```python
from build123d import *

# Parameters (mm, degrees)
F1_DEPTH = 15
F2_DEPTH = 3
F3_DEPTH = 50
F4_DEPTH = 53


with BuildPart() as f1:
    # F0 (on Top) → F1 (new body)
    with BuildSketch(Plane.XY):
        with BuildLine():
            Line((37.5, -20), (37.5, 30))
            Line((37.5, 30), (-27.5, 30))
            Line((-27.5, 30), (-27.5, 26))
            ThreePointArc((-27.5, 26), (-23.2573593129, 24.2426406871), (-21.5, 20))
            ThreePointArc((-21.5, 20), (-27.5, 14), (-33.5, 20))
            Line((-33.5, 20), (-37.5, 20))
            Line((-37.5, 20), (-37.5, -30))
            Line((-37.5, -30), (27.5, -30))
            Line((27.5, -30), (27.5, -26))
            ThreePointArc((27.5, -26), (23.2573593129, -15.7573593129), (33.5, -20))
            Line((33.5, -20), (37.5, -20))
        make_face()
        with BuildLine():
            ThreePointArc((-19, -19.25), (-27.5355339059, -22.7855339059), (-24, -14.25))
            ThreePointArc((-24, -14.25), (-20.4644660941, -15.7144660941), (-19, -19.25))
        make_face(mode=Mode.SUBTRACT)
        with BuildLine():
            ThreePointArc((25.05, -6.2), (16.5144660941, -9.7355339059), (20.05, -1.2))
            ThreePointArc((20.05, -1.2), (23.5855339059, -2.6644660941), (25.05, -6.2))
        make_face(mode=Mode.SUBTRACT)
        with BuildLine():
            ThreePointArc((5, 19.35), (3.5355339059, 15.8144660941), (0, 14.35))
            ThreePointArc((0, 14.35), (-3.5355339059, 22.8855339059), (5, 19.35))
        make_face(mode=Mode.SUBTRACT)
        with BuildLine():
            Line((-27.5, 26), (-27.5, 30))
            Line((-27.5, 30), (-37.5, 30))
            Line((-37.5, 30), (-37.5, 20))
            Line((-37.5, 20), (-33.5, 20))
            ThreePointArc((-33.5, 20), (-31.7426406871, 24.2426406871), (-27.5, 26))
        make_face()
        with BuildLine():
            Line((37.5, -30), (37.5, -20))
            Line((37.5, -20), (33.5, -20))
            ThreePointArc((33.5, -20), (31.7426406871, -24.2426406871), (27.5, -26))
            Line((27.5, -26), (27.5, -30))
            Line((27.5, -30), (37.5, -30))
        make_face()
    extrude(amount=F1_DEPTH)

    # F0 (on Top) → F2 (join)
    with BuildSketch(Plane.XY):
        with BuildLine():
            ThreePointArc((-21.5, 20), (-23.2573593129, 24.2426406871), (-27.5, 26))
            Line((-27.5, 26), (-27.5, 22))
            ThreePointArc((-27.5, 22), (-26.0857864376, 21.4142135624), (-25.5, 20))
            ThreePointArc((-25.5, 20), (-27.5, 18), (-29.5, 20))
            Line((-29.5, 20), (-33.5, 20))
            ThreePointArc((-33.5, 20), (-27.5, 14), (-21.5, 20))
        make_face()
        with BuildLine():
            Line((-27.5, 22), (-27.5, 26))
            ThreePointArc((-27.5, 26), (-31.7426406871, 24.2426406871), (-33.5, 20))
            Line((-33.5, 20), (-29.5, 20))
            ThreePointArc((-29.5, 20), (-28.9142135624, 21.4142135624), (-27.5, 22))
        make_face()
        with BuildLine():
            ThreePointArc((27.5, -26), (31.7426406871, -24.2426406871), (33.5, -20))
            Line((33.5, -20), (29.5, -20))
            ThreePointArc((29.5, -20), (28.9142135624, -21.4142135624), (27.5, -22))
            Line((27.5, -22), (27.5, -26))
        make_face()
        with BuildLine():
            Line((29.5, -20), (33.5, -20))
            ThreePointArc((33.5, -20), (23.2573593129, -15.7573593129), (27.5, -26))
            Line((27.5, -26), (27.5, -22))
            ThreePointArc((27.5, -22), (26.0857864376, -18.5857864376), (29.5, -20))
        make_face()
    extrude(amount=F2_DEPTH)

    # F0 (on Top) → F3 (join)
    with BuildSketch(Plane.XY):
        with BuildLine():
            ThreePointArc((5, 19.35), (-3.5355339059, 22.8855339059), (0, 14.35))
            ThreePointArc((0, 14.35), (3.5355339059, 15.8144660941), (5, 19.35))
        make_face()
        with BuildLine():
            ThreePointArc((2, 19.35), (1.4142135624, 17.9357864376), (0, 17.35))
            ThreePointArc((0, 17.35), (-1.4142135624, 20.7642135624), (2, 19.35))
        make_face(mode=Mode.SUBTRACT)
        with BuildLine():
            ThreePointArc((-19, -19.25), (-20.4644660941, -15.7144660941), (-24, -14.25))
            ThreePointArc((-24, -14.25), (-27.5355339059, -22.7855339059), (-19, -19.25))
        make_face()
        with BuildLine():
            ThreePointArc((-22, -19.25), (-25.4142135624, -20.6642135624), (-24, -17.25))
            ThreePointArc((-24, -17.25), (-22.5857864376, -17.8357864376), (-22, -19.25))
        make_face(mode=Mode.SUBTRACT)
        with BuildLine():
            ThreePointArc((25.05, -6.2), (23.5855339059, -2.6644660941), (20.05, -1.2))
            ThreePointArc((20.05, -1.2), (16.5144660941, -9.7355339059), (25.05, -6.2))
        make_face()
        with BuildLine():
            ThreePointArc((22.05, -6.2), (18.6357864376, -7.6142135624), (20.05, -4.2))
            ThreePointArc((20.05, -4.2), (21.4642135624, -4.7857864376), (22.05, -6.2))
        make_face(mode=Mode.SUBTRACT)
    extrude(amount=F3_DEPTH)

    # F0 (on Top) → F4 (join)
    with BuildSketch(Plane.XY):
        with BuildLine():
            ThreePointArc((2, 19.35), (-1.4142135624, 20.7642135624), (0, 17.35))
            ThreePointArc((0, 17.35), (1.4142135624, 17.9357864376), (2, 19.35))
        make_face()
        with BuildLine():
            ThreePointArc((-22, -19.25), (-22.5857864376, -17.8357864376), (-24, -17.25))
            ThreePointArc((-24, -17.25), (-25.4142135624, -20.6642135624), (-22, -19.25))
        make_face()
        with BuildLine():
            ThreePointArc((22.05, -6.2), (21.4642135624, -4.7857864376), (20.05, -4.2))
            ThreePointArc((20.05, -4.2), (18.6357864376, -7.6142135624), (22.05, -6.2))
        make_face()
    extrude(amount=F4_DEPTH)


solid = f1.part
```
CAD build for the part. Positions are in the model's coordinates, mm. A direction names the side the tool comes from. Round coordinates to 2 decimals unless told otherwise and drop trailing zeros. Loops run counter-clockwise (first coordinate to the right, second up) from the corner with the lowest first, then second, coordinate; pieces in that order, holes last. Notation, with made-up numbers: M 18,-5 L 69,-5 A11 cw 69,9 Z; hole C 59,39.25 d5. An arc over 180 degrees is marked long. Return JSON: item names as keys, results as strings. Group by question number.
(1) Tool access for faces 1 (the flat face through (-24, -19, 53)), 2 (the flat face through (-28, 17, 3)): list every direction of +Z, -Z, +X, -X, +Y, -Y with a clear straight run to the whole face (end or side of a thin tool).
(2) Saw through at A-A, the plane z = 29. List the corners of the cut face in (x, y), and give its area (3 significant figures).
(3) Saw through at B-B, the plane x = -14. List the corners of the cut face in (y, z).
(4) Drop flat-ended pins along their axis: P1, Ø1, axis at x = 0.5, z = 32.5, coming from the -Y side; P2, Ø3.5, axis at x = -27, y = 21.5, coming from the +Z side; P3, Ø10, axis at x = 26, y = -21.5, coming from the +Z side; P4, Ø2.5, axis at x = 27.5, y = -20, coming from the -Z side. Give the stop position or say it passes through.
(5) Saw through at C-C, the plane y = 2. List the corners of the cut face in (x, z).
(6) Wall check: probe 1 along Y at (x, z) = (27.5, 1.95); probe 2 along X at (y, z) = (-20, 9); probe 3 along X at (y, z) = (-20, 2.3). Give the ranges that are in metal, low to high. Write a range as [from, to].
Answer list:
{
 "1": {"face 1": "+Z, +X, -X, +Y, -Y", "face 2": "+Z"},
 "2": {"outline": "C -24,-19.25 d10; C 0,19.35 d10; C 20.05,-6.2 d10", "area": "236 mm2"},
 "3": {"outline": "M -30,0 L 30,0 L 30,15 L -30,15 Z"},
 "4": {"P1": "y = 14.35", "P2": "z = 3", "P3": "z = 15", "P4": "through"},
 "5": {"outline": "M -37.5,0 L 37.5,0 L 37.5,15 L -37.5,15 Z"},
 "6": {"probe 1": "[-30, -22], [-18, 30]", "probe 2": "[-37.5, 21.5], [33.5, 37.5]", "probe 3": "[-37.5, 25.5], [29.5, 37.5]"}
}
